Part model, mm, in its own coordinate system. A direction names the side the tool comes from. Coordinates: 2 decimals unless noted, no trailing zeros. Order: outer loops, then holes, each group sorted by start corner. A loop starts at its lowest first (then second) coordinate and runs counter-clockwise, first axis right, second up.
from build123d import *

# Parameters (mm, degrees)
SKETCH_1_W                = 40
SKETCH_1_H                = 34
EXTRUDE_1_DEPTH           = 12.5
HOLE_WIZARD_1_D           = 3.4
HOLE_WIZARD_1_CBORE_D     = 6
HOLE_WIZARD_1_CBORE_DEPTH = 38
SKETCH_2_W                = 35
SKETCH_2_H                = 5
CUT_EXTRUDE_1_DEPTH       = 37.249137921
HOLE_WIZARD_M2_5_1_D      = 2.05
HOLE_WIZARD_M2_5_1_DEPTH  = 6
HOLE_WIZARD_M5_1_D        = 4.2
HOLE_WIZARD_1_2_REACH     = 39.38
HOLE_WIZARD_1_2_BORE_R    = 3
HOLE_WIZARD_2_D           = 4.2


with BuildPart() as part:
    # 草图1 → 凸台-拉伸1 (new, symmetric)
    with BuildSketch(Plane.XY):
        Rectangle(SKETCH_1_W, SKETCH_1_H)
    extrude(amount=EXTRUDE_1_DEPTH, both=True)

    # Hole Wizard 1 (through all)
    with Locations(Plane(origin=(20, -11.097573199, 8.576816528), x_dir=(0, 0, -1), z_dir=(1, 0, 0))):
        with Locations((1.076816528, 24.097573199), (16.076816528, 24.097573199)):
            CounterBoreHole(HOLE_WIZARD_1_D / 2, HOLE_WIZARD_1_CBORE_D / 2, HOLE_WIZARD_1_CBORE_DEPTH)

    # 草图2 → 切除-拉伸1 (cut, through all)
    with BuildSketch(Plane.XY.offset(12.5)):
        with Locations((2.5, 14.5)):
            Rectangle(SKETCH_2_W, SKETCH_2_H)
        Polygon((-20, -17), (2, -17), (2, -11), (10, -11), (10, 7.7), (-20, 7.7), align=None)
    extrude(amount=-CUT_EXTRUDE_1_DEPTH, mode=Mode.SUBTRACT)

    # M2.5 螺纹孔1
    with Locations(Plane(origin=(23.183007196, -11, -17.133988824), x_dir=(0, 0, -1), z_dir=(0, 1, 0))):
        with Locations((-21.133988824, 17.183007196)):
            Hole(HOLE_WIZARD_M2_5_1_D / 2, depth=HOLE_WIZARD_M2_5_1_DEPTH)

    # M5 螺纹孔1 (through all)
    with Locations(Plane(origin=(20, 0, 0), x_dir=(0, 0, -1), z_dir=(1, 0, 0))):
        with Locations((0, 2), (-9, -0.7)):
            Hole(HOLE_WIZARD_M5_1_D / 2)

    # Hole Wizard 1 2 bore → Hole Wizard 1 2 (cut, up to next)
    with BuildSketch(Plane(origin=(0, 12, 0), x_dir=(1, 0, 0), z_dir=(0, 1, 0)), mode=Mode.PRIVATE) as hole_wizard_1_2_sk1:
        with Locations((6, -4)):
            Circle(HOLE_WIZARD_1_2_BORE_R)
    hole_wizard_1_2_tool1 = extrude(hole_wizard_1_2_sk1.sketch, amount=-HOLE_WIZARD_1_2_REACH, mode=Mode.PRIVATE) & part.part
    add(hole_wizard_1_2_tool1.solids().sort_by_distance((6, 12, 4))[0], mode=Mode.SUBTRACT)

    # 孔2 (through all)
    with Locations(Plane(origin=(20, 0, 0), x_dir=(0, 0, -1), z_dir=(1, 0, 0))):
        with Locations((7.5, 0.2)):
            Hole(HOLE_WIZARD_2_D / 2)


solid = part.part
Q1. Cut at B-B on z = -7.5. Write the cut outline in (x, y), and give its area (3 significant figures).
Results list:
outline: (-20, 7.7) - (10, 7.7) - (10, 2.3) - (20, 2.3) - (20, 10) - (-18, 10) - (-18, 11.3) - (-20, 11.3) - close; (-20, 14.7) - (-18, 14.7) - (-18, 16) - (-15, 16) - (-15, 17) - (-20, 17) - close; (2, -17) - (20, -17) - (20, -1.9) - (10, -1.9) - (10, -11) - (2, -11) - close
area: 355 mm2
Q2. Cut at A-A on z = 0. Write the cut outline in (x, y).
Results list:
outline: (-20, 7.7) - (10, 7.7) - (10, 4.1) - (20, 4.1) - (20, 12) - (-15, 12) - (-15, 17) - (-20, 17) - close; (2, -17) - (20, -17) - (20, -0.1) - (10, -0.1) - (10, -11) - (2, -11) - close
Q3. Which spindle directions (+Z, -Z, +X, -X, +Y, -Y) get a long thin tool onto all of the face, cutting with end or side? Do faces 5 (the face through (6, 9, 1)), 6 (the face through (-18, 11, 8)), 7 (the face through (2, 12, 11)), 8 (the face through (6, -11, 0)). Say none if no direction does.
Results list:
face 5: +Y
face 6: +X
face 7: +Z, -Z, +X, +Y
face 8: +Z, -Z, -X
Q4. Wall check: line 1 along Y through (x, z) = (13.75, 0); line 2 along Z through (x, y) = (6, 9); line 3 along Y through (x, z) = (17.25, -7.5). Give the ranges that are in metal, low to high.
Results list:
line 1: y = -17 to -0.1, 4.1 to 12
line 2: z = -12.5 to 1, 7 to 12.5
line 3: y = -17 to -1.9, 2.3 to 10
Q5. Pin check, flat tips, straight feed: pin 1 Ø1.1 at (x, z) = (8, -11) entering from +Y; pin 2 Ø3.5 at (y, z) = (0.2, -7.5) entering from -X; pin 3 Ø10 at (y, z) = (-12.5, 1.5) entering from -X; pin 4 Ø15 at (y, z) = (0, -2) entering from -X. Stop position of each tip, or through.
Results list:
pin 1: stops at y = 12
pin 2: passes through
pin 3: stops at x = 2
pin 4: stops at x = 10
Q6. Cut at C-C on x = 14.5. Write the cut outline in (y, z).
Results list:
outline: (-17, -12.5) - (12, -12.5) - (12, -10.33) arc R3 cw to (12, -4.67) - (12, 4.67) arc R3 cw to (12, 10.33) - (12, 12.5) - (-17, 12.5) - close; hole circle Ø4.2 at (-0.7, 9); hole circle Ø4.2 at (0.2, -7.5); hole circle Ø4.2 at (2, 0)
Q7. Mould opens along Y. For faces 1 (the face through (10, -2, 0)), 2 (the face through (-19.01, 13.07, -9.2)), 3 (the face through (-15, 15, 0)), 4 (the face through (11, -17, 0)) say: pulls with the +Y half, pulls with the -Y half, needs draft (parallel to the pull), parting line crosses it, or undercut.
Results list:
face 1: undercut
face 2: undercut
face 3: needs draft
face 4: pulls with the -Y half
Q8. Cut at D-D on y = 13. Write the cut outline in (x, z).
Results list:
outline: (-20, -12.5) - (-15, -12.5) - (-15, -10.5) - (-18, -10.5) - (-18, -9.2) - (-20, -9.2) - close; (-20, -5.8) - (-18, -5.8) - (-18, -4.5) - (-15, -4.5) - (-15, 4.5) - (-18, 4.5) - (-18, 5.8) - (-20, 5.8) - close; (-20, 9.2) - (-18, 9.2) - (-18, 10.5) - (-15, 10.5) - (-15, 12.5) - (-20, 12.5) - close
